from build123d import *

# Parameters (mm, degrees)
SKETCH2_W                 = 29.5
SKETCH2_H                 = 10.8
SKETCH2_W_2               = 12
SKETCH2_H_2               = 2
F_2_0MM_DOWEL_HOLE1_D     = 2
F_2_0MM_DOWEL_HOLE1_DEPTH = 0.4
F_2_0MM_DOWEL_HOLE1_TIP   = 0.600860619


with BuildPart() as part:
    # Sketch2 → Revolve1 (revolve)
    with BuildSketch(Plane.XY, mode=Mode.PRIVATE) as revolve1_sk:
        Polygon((0, -10.8), (0, 0), (-18, 0), (-18, -7), (-18, -11), (0, -11), align=None)
        with Locations((14.75, -5.4)):
            Rectangle(SKETCH2_W, SKETCH2_H)
        Polygon((-18, -7), (-18, 0), (-20, 0), (-20, -2), (-20, -7), align=None)
        with Locations((-26, -1)):
            Rectangle(SKETCH2_W_2, SKETCH2_H_2)
    revolve(revolve1_sk.sketch.rotate(Axis((0, 0, 0), (-1, 0, 0)), 180), axis=Axis((0, 0, 0), (-1, 0, 0)))

    # Ø2.0mm Dowel Hole1
    with Locations(Plane.ZY.offset(18)):
        with Locations((-9, 0), (0, 9), (9, 0), (0, -9)):
            Hole(F_2_0MM_DOWEL_HOLE1_D / 2, depth=F_2_0MM_DOWEL_HOLE1_DEPTH)
            with Locations((0, 0, -(F_2_0MM_DOWEL_HOLE1_DEPTH + F_2_0MM_DOWEL_HOLE1_TIP / 2))):  # 118° drill point
                Cone(0, F_2_0MM_DOWEL_HOLE1_D / 2, F_2_0MM_DOWEL_HOLE1_TIP, mode=Mode.SUBTRACT)


solid = part.part
CAD build for the part. Positions are in the model's coordinates, mm. A direction names the side the tool comes from. Round coordinates to 2 decimals unless told otherwise and drop trailing zeros. Write each loop counter-clockwise with the first axis right and the second up, starting at its lowest first coordinate (ties: lowest second). Pieces come first, ordered by that corner, then holes.
(1) Mould opens along Z. For faces 1 (the face through (-17.8, 9.99, 0.13)), 2 (the face through (-17, 0, 9)), 3 (the face through (-18, -7.2, -0.2)), 4 (the face through (-8.87, -2.38, 10.74)) say: pulls with the +Z half, pulls with the -Z half, needs draft (parallel to the pull), parting line crosses it, or undercut.
(2) Slice it at C-C, the plane x = -12. Write the cut outline in (y, z).
(3) Drop flat-ended pins along their axis: P1, Ø3, axis at y = 0, z = -9, coming from the -X side; P2, Ø8, axis at x = 10, y = -3, coming from the +Z side; P3, Ø5, axis at x = -13.5, y = 5, coming from the -Z side. Give the stop position or say it passes through.
(4) Slice it at B-B, the plane x = 9. Write the cut outline in (y, z).
(5) Probe line 1 along Z through (x, y) = (-17.7, 0); line 2 along X through (y, z) = (-2.5, -9.75); line 3 along X through (y, z) = (-6.75, 1.5). List the from-to ranges inside material, lowest first.
(6) 3-axis set-ups, long thin cutter, end or side, ignore diameter. For faces 5 (the face through (-26, 0, 2)), 6 (the face through (14.96, -8.57, 6.57)), 7 (the face through (29.5, 0, 0)): which of +Z, -Z, +X, -X, +Y, -Y reach the whole face in a straight line?
(7) Slice it at A-A, the plane y = 3.5. Write the cut outline in (x, z), and give its area (3 significant figures).
From the geometry:
1. face 1: undercut
1. face 2: undercut
1. face 3: needs draft
1. face 4: parting line crosses it
2. outline: circle Ø22 at (0, 0)
3. P1: stops at x = -18
3. P2: stops at z = 10.8
3. P3: stops at z = -10.71
4. outline: circle Ø21.6 at (0, 0)
5. line 1: z = -11 to -10, -8 to 8, 10 to 11
5. line 2: x = -18 to 29.5
5. line 3: x = -20 to 29.5
6. face 5: -X
6. face 6: +X
6. face 7: +Z, -Z, +X, +Y, -Y
7. outline: (-20, -6.06) - (-18, -6.06) - (-18, -10.43) - (0, -10.43) - (0, -10.22) - (29.5, -10.22) - (29.5, 10.22) - (0, 10.22) - (0, 10.43) - (-18, 10.43) - (-18, 6.06) - (-20, 6.06) - close
7. area: 1,000 mm2
